from build123d import *

# Parameters (mm, degrees)
SKETCH1_W           = 50.8
SKETCH1_H           = 15.24
BOSS_EXTRUDE1_DEPTH = 5.08
CUT_EXTRUDE2_REACH  = 7.08
SKETCH3_W           = 10.16
SKETCH3_H           = 5.08
CUT_EXTRUDE3_REACH  = 7.08
SKETCH4_W           = 10.16
SKETCH4_H           = 5.08


with BuildPart() as part:
    # Sketch1 → Boss-Extrude1 (new body)
    with BuildSketch(Plane.XY):
        with Locations((25.4, 7.62)):
            Rectangle(SKETCH1_W, SKETCH1_H)
    extrude(amount=BOSS_EXTRUDE1_DEPTH)

    # Sketch3 → Cut-Extrude2 (cut, up to next)
    with BuildSketch(Plane(origin=(0, 0, 0), x_dir=(-1, 0, 0), z_dir=(0, 0, -1)), mode=Mode.PRIVATE) as cut_extrude2_sk1:
        with Locations((-5.08, 2.54)):
            Rectangle(SKETCH3_W, SKETCH3_H)
    cut_extrude2_tool1 = extrude(cut_extrude2_sk1.sketch, amount=-CUT_EXTRUDE2_REACH, mode=Mode.PRIVATE) & part.part
    add(cut_extrude2_tool1.solids().sort_by_distance((5.08, 2.54, 0))[0], mode=Mode.SUBTRACT)
    # Sketch3 → Cut-Extrude2 (cut, up to next)
    with BuildSketch(Plane(origin=(0, 0, 0), x_dir=(-1, 0, 0), z_dir=(0, 0, -1)), mode=Mode.PRIVATE) as cut_extrude2_sk2:
        with Locations((-25.4, 2.54)):
            Rectangle(SKETCH3_W, SKETCH3_H)
    cut_extrude2_tool2 = extrude(cut_extrude2_sk2.sketch, amount=-CUT_EXTRUDE2_REACH, mode=Mode.PRIVATE) & part.part
    add(cut_extrude2_tool2.solids().sort_by_distance((25.4, 2.54, 0))[0], mode=Mode.SUBTRACT)
    # Sketch3 → Cut-Extrude2 (cut, up to next)
    with BuildSketch(Plane(origin=(0, 0, 0), x_dir=(-1, 0, 0), z_dir=(0, 0, -1)), mode=Mode.PRIVATE) as cut_extrude2_sk3:
        with Locations((-45.72, 2.54)):
            Rectangle(SKETCH3_W, SKETCH3_H)
    cut_extrude2_tool3 = extrude(cut_extrude2_sk3.sketch, amount=-CUT_EXTRUDE2_REACH, mode=Mode.PRIVATE) & part.part
    add(cut_extrude2_tool3.solids().sort_by_distance((45.72, 2.54, 0))[0], mode=Mode.SUBTRACT)

    # Sketch4 → Cut-Extrude3 (cut, up to next)
    with BuildSketch(Plane.XY.offset(5.08), mode=Mode.PRIVATE) as cut_extrude3_sk1:
        with Locations((15.24, 12.7)):
            Rectangle(SKETCH4_W, SKETCH4_H)
    cut_extrude3_tool1 = extrude(cut_extrude3_sk1.sketch, amount=-CUT_EXTRUDE3_REACH, mode=Mode.PRIVATE) & part.part
    add(cut_extrude3_tool1.solids().sort_by_distance((15.24, 12.7, 5.08))[0], mode=Mode.SUBTRACT)
    # Sketch4 → Cut-Extrude3 (cut, up to next)
    with BuildSketch(Plane.XY.offset(5.08), mode=Mode.PRIVATE) as cut_extrude3_sk2:
        with Locations((35.56, 12.7)):
            Rectangle(SKETCH4_W, SKETCH4_H)
    cut_extrude3_tool2 = extrude(cut_extrude3_sk2.sketch, amount=-CUT_EXTRUDE3_REACH, mode=Mode.PRIVATE) & part.part
    add(cut_extrude3_tool2.solids().sort_by_distance((35.56, 12.7, 5.08))[0], mode=Mode.SUBTRACT)


solid = part.part
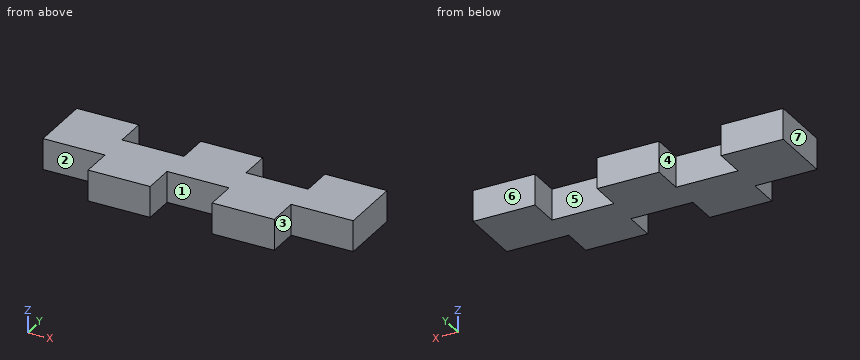
Verification items for the finished model (mm, model axes). Face numbers are marked on the shaded views. A direction names the side the tool comes from. Coordinates: 2 decimals unless noted, no trailing zeros. Order: outer loops, then holes, each group sorted by start corner. A loop starts at its lowest first (then second) coordinate and runs counter-clockwise, first axis right, second up. Notation, with made-up numbers: (-7.75, -37) -> (44.25, -37) arc R20 cw to (44.25, -15) -> close; hole circle Ø5 at (8, 34). An arc over 180 degrees is marked (long way). Use CSV: the item, a comma, the result in double quotes. Start each with the question number.
Q1. Section check B-B, the plane y = 12.5. Record the cut outline in (x, z), and give its area (3 significant figures).
Q2. Draft check along X on the marked faces 5, 6 and 7. Enter one of: +X half, -X half, draft (parallel to the pull), parting line (faces both ways), or undercut.
Q3. Tool access check on the marked faces 1, 2, 3 and 4. Record the directions out of +Z, -Z, +X, -X, +Y, -Y that give a thin tool (end or side, any length) a straight path to the whole face; none if there is none.
Q4. Section check D-D, the plane x = 26. Record the cut outline in (y, z), and give its area (3 significant figures).
Q5. Section check A-A, the plane y = 4.5. Record the cut outline in (x, z).
Q6. Depth check by flat-ended pin: P1, Ø1.5, axis at x = 27.5, z = 3, coming from the -Y side; P2, Ø1.5, axis at x = 34, z = 2, coming from the +Y side. Enter the tip coordinate at first touch or a pass-through.
Q7. Section check C-C, the plane z = 4.65. Record the cut outline in (x, y), and give its area (3 significant figures).
Q8. Thickness scan on line 1 along X through (y, z) = (12, 1.5); line 2 along X through (y, z) = (2.25, 2.8); line 3 along Y through (x, z) = (46, 0.9). Record the ranges inside material, lowest first.
Returned:
1,outline,"(0, 0) -> (10.16, 0) -> (10.16, 5.08) -> (0, 5.08) -> close; (20.32, 0) -> (30.48, 0) -> (30.48, 5.08) -> (20.32, 5.08) -> close; (40.64, 0) -> (50.8, 0) -> (50.8, 5.08) -> (40.64, 5.08) -> close"
1,area,"155 mm^2"
2,face 5,"undercut"
2,face 6,"draft"
2,face 7,"-X half"
3,face 1,"+Z, -Z, -Y"
3,face 2,"+Z, -Z, -X, -Y"
3,face 3,"+Z, -Z, +X, -Y"
3,face 4,"+Z, -Z, +Y"
4,outline,"(5.08, 0) -> (15.24, 0) -> (15.24, 5.08) -> (5.08, 5.08) -> close"
4,area,"51.6 mm^2"
5,outline,"(10.16, 0) -> (20.32, 0) -> (20.32, 5.08) -> (10.16, 5.08) -> close; (30.48, 0) -> (40.64, 0) -> (40.64, 5.08) -> (30.48, 5.08) -> close"
6,P1,"stops at y = 5.08"
6,P2,"stops at y = 10.16"
7,outline,"(0, 5.08) -> (10.16, 5.08) -> (10.16, 0) -> (20.32, 0) -> (20.32, 5.08) -> (30.48, 5.08) -> (30.48, 0) -> (40.64, 0) -> (40.64, 5.08) -> (50.8, 5.08) -> (50.8, 15.24) -> (40.64, 15.24) -> (40.64, 10.16) -> (30.48, 10.16) -> (30.48, 15.24) -> (20.32, 15.24) -> (20.32, 10.16) -> (10.16, 10.16) -> (10.16, 15.24) -> (0, 15.24) -> close"
7,area,"516 mm^2"
8,line 1,"x = 0 to 10.16, 20.32 to 30.48, 40.64 to 50.8"
8,line 2,"x = 10.16 to 20.32, 30.48 to 40.64"
8,line 3,"y = 5.08 to 15.24"
